CAD build for the part. Positions are in the model's coordinates, mm. Face numbers are marked on the shaded views. Round coordinates to 2 decimals unless told otherwise and drop trailing zeros. Order: outer loops, then holes, each group sorted by start corner. A loop starts at its lowest first (then second) coordinate and runs counter-clockwise, first axis right, second up. Notation, with made-up numbers: M 33,-38 L 82,-38 A9 ccw 82,-29 Z; hole C 67,2 d3. An arc over 180 degrees is marked long. Answer as a JSON object with one key per item and string values. Group by question number.
Autodesk Inventor part; units mm, degrees
ref_plane "YZ Plane" through (0, 0, 0) normal (1, 0, 0) x (0, 1, 0)
ref_plane "XZ Plane" through (0, 0, 0) normal (0, 1, 0) x (-1, 0, 0)
ref_plane "XY Plane" through (0, 0, 0) normal (0, 0, 1) x (1, 0, 0)
sketch "Sketch1" plane through (0, 0, 0) normal (0, 1, 0) x (-1, 0, 0)
  line L0 (7.0148, -0.75) -> (4.1569, -5.7)
  line L1 (2.8579, -6.45) -> (-2.8579, -6.45)
  line L2 (-4.1569, -5.7) -> (-7.0148, -0.75)
  line L3 (-7.0148, 0.75) -> (-4.1569, 5.7)
  line L4 (-2.8579, 6.45) -> (2.8579, 6.45)
  line L5 (4.1569, 5.7) -> (7.0148, 0.75)
  arc A0 (7.0148, -0.75) -> (7.0148, 0.75) centre (5.7158, 0) ccw
  arc A1 (4.1569, 5.7) -> (2.8579, 6.45) centre (2.8579, 4.95) ccw
  arc A2 (-2.8579, 6.45) -> (-4.1569, 5.7) centre (-2.8579, 4.95) ccw
  arc A3 (-7.0148, 0.75) -> (-7.0148, -0.75) centre (-5.7158, 0) ccw
  arc A4 (-4.1569, -5.7) -> (-2.8579, -6.45) centre (-2.8579, -4.95) ccw
  arc A5 (2.8579, -6.45) -> (4.1569, -5.7) centre (2.8579, -4.95) ccw
  circle A6 centre (0, 0) radius 3.8
  point P0 (7.4478, 0)
  point P1 (3.7239, -6.45)
  point P2 (-3.7239, -6.45)
  point P3 (-7.4478, 0)
  point P4 (-3.7239, 6.45)
  point P5 (3.7239, 6.45)
  dimension "d0" = 12.9
  dimension "d1" = 1.5
  dimension "d2" = 1.5
  dimension "d3" = 7.6
extrude "Extrusion1" add sketch "Sketch1" along normal blind 2.5
fillet "Fillet1" radius 0.5 24 edges at (3.6079, 2.5, 6.249) (5.5859, 2.5, 3.225) (7.2158, 2.5, 0) (5.5859, 2.5, -3.225) (3.6079, 2.5, -6.249) (0, 2.5, -6.45) (-3.6079, 2.5, -6.249) (-5.5859, 2.5, -3.225) (-7.2158, 2.5, 0) (-5.5859, 2.5, 3.225) (-3.6079, 2.5, 6.249) (0, 2.5, 6.45) (3.6079, 0, 6.249) (5.5859, 0, 3.225) (7.2158, 0, 0) (5.5859, 0, -3.225) (3.6079, 0, -6.249) (0, 0, -6.45) (-3.6079, 0, -6.249) (-5.5859, 0, -3.225) (-7.2158, 0, 0) (-5.5859, 0, 3.225) (-3.6079, 0, 6.249) (0, 0, 6.45)
thread "Thread1"
properties part number "LED Nut"
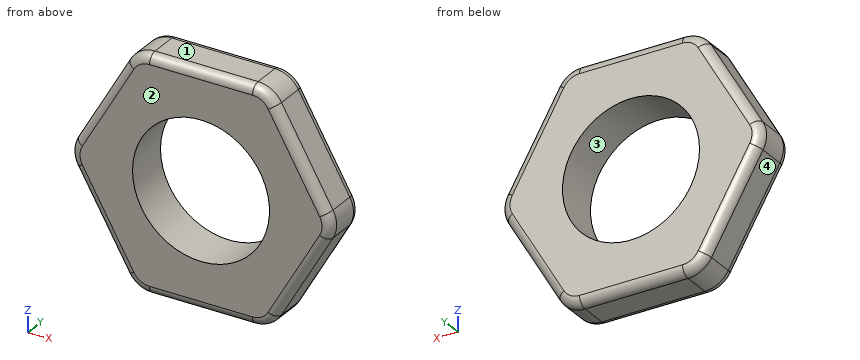
Item 1: Drill centre lines: line 1 (Z direction, x = 0, y = 1.45); line 2 (Z direction, x = 0.75, y = 1.75); line 3 (X direction, y = 1.6, z = -1.25). Where is each one in solid material? Low to high. Write a range as [from, to].
Item 2: Two-plate mould, pull along Z, no slides. Class the marked faces 1, 2, 3 and 4: +Z half, -Z half, draft (parallel to the pull), parting line (faces both ways), or undercut.
Item 3: Cut at B-B, the plane y = 1.8. Give the cut face in (x, z), and give its area (3 significant figures).
Item 4: Cut at A-A, the plane z = 0. Give the cut face in (x, y), and give its area (3 significant figures).
Item 5: Cut at C-C, the plane x = 0. Give the cut face in (y, z), and give its area (3 significant figures).
Response values:
{
 "1": {"line 1": "[-6.45, -3.8], [3.8, 6.45]", "line 2": "[-6.45, -3.73], [3.73, 6.45]", "line 3": "[-6.73, -3.59], [3.59, 6.73]"},
 "2": {"face 1": "+Z half", "face 2": "draft", "face 3": "undercut", "face 4": "-Z half"},
 "3": {"outline": "M -7.01,-0.75 L -4.16,-5.7 A1.5 ccw -2.86,-6.45 L 2.86,-6.45 A1.5 ccw 4.16,-5.7 L 7.01,-0.75 A1.5 ccw 7.01,0.75 L 4.16,5.7 A1.5 ccw 2.86,6.45 L -2.86,6.45 A1.5 ccw -4.16,5.7 L -7.01,0.75 A1.5 ccw Z; hole C 0,0 d7.6", "area": "98.0 mm^2"},
 "4": {"outline": "M -7.22,0.5 A0.5 ccw -6.72,0 L -3.8,0 L -3.8,2.5 L -6.72,2.5 A0.5 ccw -7.22,2 Z; M 3.8,0 L 6.72,0 A0.5 ccw 7.22,0.5 L 7.22,2 A0.5 ccw 6.72,2.5 L 3.8,2.5 Z", "area": "16.9 mm^2"},
 "5": {"outline": "M 0,-5.95 A0.5 ccw 0.5,-6.45 L 2,-6.45 A0.5 ccw 2.5,-5.95 L 2.5,-3.8 L 0,-3.8 Z; M 0,3.8 L 2.5,3.8 L 2.5,5.95 A0.5 ccw 2,6.45 L 0.5,6.45 A0.5 ccw 0,5.95 Z", "area": "13.0 mm^2"}
}
